Part model, mm, in its own coordinate system. Round coordinates to 2 decimals unless told otherwise and drop trailing zeros. Order: outer loops, then holes, each group sorted by start corner. A loop starts at its lowest first (then second) coordinate and runs counter-clockwise, first axis right, second up. Notation, with made-up numbers: (83, -4.5) - (117, -4.5) arc R32 ccw to (117, 21.5) - close; hole circle Ø11 at (-12.75, 66.5). An arc over 180 degrees is marked (long way). Return JSON: item names as keys, results as strings. Group by question number.
Item 1: Probe probe 1 along X at (y, z) = (-68.5, 2); probe 2 along X at (y, z) = (-132, -0.25); probe 3 along Z at (x, y) = (16, -84.5). List the from-to ranges inside material, lowest first.
Item 2: Drop flat-ended pins along their axis: pin 1 (2 mm diameter, centred on x = 14.5, y = -104, fed in from +Z); pin 2 (1.5 mm diameter, centred on y = -50.5, z = -1, fed in from +X); pin 3 (4 mm diameter, centred on x = 14, y = -116.5, fed in from +Z) (3 decimals). Give the stop position or say it passes through.
Item 3: Saw through at C-C on x = 12. List the corners of the cut face in (y, z).
Item 4: Saw through at B-B on z = 1.75. List the corners of the cut face in (x, y), and give its area (3 significant figures).
Item 5: Saw through at A-A on y = -105. List the corners of the cut face in (x, z), and give its area (3 significant figures).
```python
from build123d import *

# Parameters (mm, degrees)
F1_DEPTH = 152.4


# Not quite as in the source:
# - ends of sketch curves that miss each other by under 0.0002 mm in the source are joined


with BuildPart() as f1:
    # F0 (on Front) → F1 (new body)
    with BuildSketch(Plane.XZ):
        with BuildLine():
            ThreePointArc((14.7938744, 0.7382764), (12.0081110559, 1.3810143829), (9.7855278, 3.1792672))
            Line((9.7855278, 3.1792672), (-20.665186, 3.1792672))
            Line((-20.665186, 3.1792672), (-20.665186, -3.1792672))
            Line((-20.665186, -3.1792672), (20.6652114, -3.1792672))
            ThreePointArc((20.6652114, -3.1792672), (18.3230324667, -0.331016316), (14.7938744, 0.7382764))
        make_face()
    extrude(amount=F1_DEPTH)


solid = f1.part
```
Filled in:
{
 "1": {"probe 1": "x = -20.67 to 10.99", "probe 2": "x = -20.67 to 18.2", "probe 3": "z = -3.18 to 0.62"},
 "2": {"pin 1": "stops at z = 0.87", "pin 2": "stops at x = 19.84", "pin 3": "stops at z = 1.385"},
 "3": {"outline": "(-152.4, -3.18) - (0, -3.18) - (0, 1.38) - (-152.4, 1.38) - close"},
 "4": {"outline": "(-20.67, -152.4) - (11.35, -152.4) - (11.35, 0) - (-20.67, 0) - close", "area": "4,880 mm^2"},
 "5": {"outline": "(-20.67, -3.18) - (20.67, -3.18) arc R6.36 ccw to (14.79, 0.74) arc R6.36 cw to (9.79, 3.18) - (-20.67, 3.18) - close", "area": "234 mm^2"}
}
